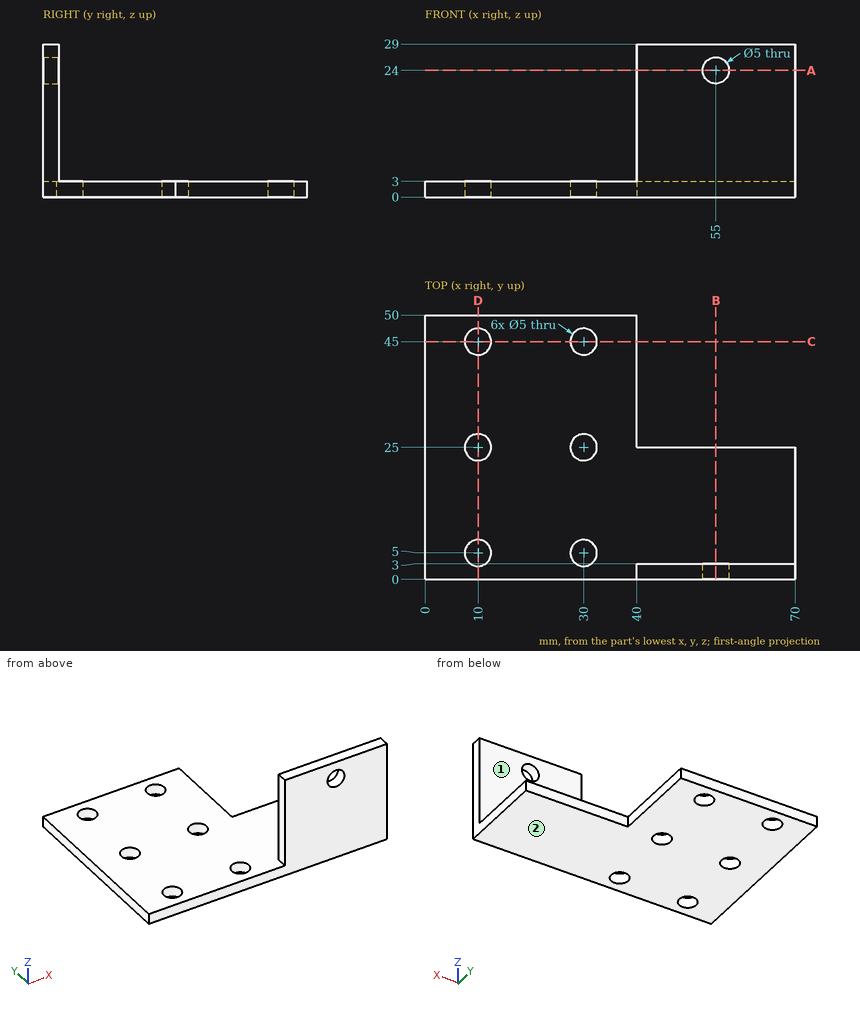
The drawing under review shows one solid part. Ordinate dimensions are in mm from its lowest x, y, z. A direction names the side the tool comes from. Round coordinates to 2 decimals unless told otherwise and drop trailing zeros. Write each loop counter-clockwise with the first axis right and the second up, starting at its lowest first coordinate (ties: lowest second). Pieces come first, ordered by that corner, then holes. Notation, with made-up numbers: (35.25, -34.75) -> (89.25, -34.75) arc R34 cw to (89.25, 0.25) -> close; hole circle Ø11 at (-18, -32.75). An arc over 180 degrees is marked (long way). One line per question, with ' | ' between items.
(1) Take a section at A-A, the plane z = 24. State the section outline as (x, y) points.
Result sheet:
outline: (40, 0) -> (52.5, 0) -> (52.5, 3) -> (40, 3) -> close; (57.5, 0) -> (70, 0) -> (70, 3) -> (57.5, 3) -> close
(2) Insertion check: P1, Ø3.5, axis at y = 33.5, z = 2, coming from the +X side; P2, Ø4, axis at x = 37.5, z = 20.5, coming from the -Y side; P3, Ø2.5, axis at y = 1, z = 16, coming from the -X side; P4, Ø8, axis at x = 30, y = 45, coming from the +Z side. Each pin has a flat end and moves straight along its axis. Give the tip position at first contact, or say it passes through.
Result sheet:
P1: x = 40 | P2: through | P3: x = 40 | P4: z = 3
(3) Take a section at B-B, the plane x = 55. State the section outline as (y, z) points, and give its area (3 significant figures).
Result sheet:
outline: (0, 0) -> (25, 0) -> (25, 3) -> (3, 3) -> (3, 21.5) -> (0, 21.5) -> close; (0, 26.5) -> (3, 26.5) -> (3, 29) -> (0, 29) -> close | area: 138 mm2
(4) Take a section at C-C, the plane y = 45. State the section outline as (x, z) points, and give its area (3 significant figures).
Result sheet:
outline: (0, 0) -> (7.5, 0) -> (7.5, 3) -> (0, 3) -> close; (12.5, 0) -> (27.5, 0) -> (27.5, 3) -> (12.5, 3) -> close; (32.5, 0) -> (40, 0) -> (40, 3) -> (32.5, 3) -> close | area: 90.0 mm2
(5) Machinability: for the marked faces 1 and 2, which of the approach directions +Z, -Z, +X, -X, +Y, -Y give a long, thin tool a straight path to every point of the face, cutting with its end or side? Answer none if there is none.
Result sheet:
face 1: +Z, +X, -X, +Y | face 2: -Z, +X, -X, +Y, -Y
(6) Wall thickness on line 1 (X direction, y = 2.15, z = 24); line 2 (Y direction, x = 30, z = 1.7); line 3 (Y direction, x = 53, z = 13.25): over which ranges is each line inside the solid? List them lowest first. Write a range as [from, to].
Result sheet:
line 1: [40, 52.5], [57.5, 70] | line 2: [0, 2.5], [7.5, 22.5], [27.5, 42.5], [47.5, 50] | line 3: [0, 3]
(7) Take a section at D-D, the plane x = 10. State the section outline as (y, z) points.
Result sheet:
outline: (0, 0) -> (2.5, 0) -> (2.5, 3) -> (0, 3) -> close; (7.5, 0) -> (22.5, 0) -> (22.5, 3) -> (7.5, 3) -> close; (27.5, 0) -> (42.5, 0) -> (42.5, 3) -> (27.5, 3) -> close; (47.5, 0) -> (50, 0) -> (50, 3) -> (47.5, 3) -> close
